Read the model definition and answer for the solid it produces. Units are mm, in the model's axes. A direction names the side the tool comes from. Coordinates: 2 decimals unless noted, no trailing zeros. Write each loop counter-clockwise with the first axis right and the second up, starting at its lowest first coordinate (ties: lowest second). Pieces come first, ordered by that corner, then holes. Notation, with made-up numbers: (87.5, 54.5) -> (111.5, 54.5) arc R36 cw to (111.5, 90.5) -> close; hole circle Ø2 at (67.5, -32.75). An arc over 180 degrees is marked (long way). Use CSV: the item, a comma, the result in double quotes. Start each with the question number.
Autodesk Inventor part; units mm, degrees
ref_plane "YZ Plane" through (0, 0, 0) normal (1, 0, 0) x (0, 1, 0)
ref_plane "XZ Plane" through (0, 0, 0) normal (0, 1, 0) x (-1, 0, 0)
ref_plane "XY Plane" through (0, 0, 0) normal (0, 0, 1) x (1, 0, 0)
sketch "Sketch2" plane through (0, 0, 0) normal (0, 0, 1) x (1, 0, 0)
  circle A0 centre (0, 0) radius 12.7
  dimension "d4" = 25.4
extrude "Extrusion2" add sketch "Sketch2" against normal blind 25.4
chamfer "Chamfer1" distance 1.524 angle 45 1 edges at (-12.7, 0, 0) measured on face at (-3.6254, -0.9542, 0)
sketch "Sketch3" plane through (0, 0, -25.4) normal (0, 0, -1) x (-1, 0, 0)
  circle A0 centre (0, 0) radius 9.144
  dimension "d10" = 18.288
extrude "Extrusion3" add sketch "Sketch3" along normal blind 6.35
sketch "Sketch4" plane through (0, 0, -31.75) normal (0, 0, -1) x (-1, 0, 0)
  circle A0 centre (0, 0) radius 11.049
  dimension "d13" = 22.098
extrude "Extrusion4" add sketch "Sketch4" along normal blind 25.4
thread "Thread1"
chamfer "Chamfer2" distance 1.524 angle 45 1 edges at (11.049, 0, -57.15) measured on face at (-0.3422, 2.8186, -57.15)
sketch "Sketch5" plane through (0, 0, -57.15) normal (0, 0, -1) x (-1, 0, 0)
  circle A0 centre (0, 0) radius 6.477
  dimension "d21" = 12.954
extrude "Extrusion5" add sketch "Sketch5" along normal blind 6.35
sketch "Sketch6" plane through (0, 0, -63.5) normal (0, 0, -1) x (-1, 0, 0)
  circle A0 centre (0, 0) radius 7.874
  dimension "d24" = 15.748
extrude "Extrusion6" add sketch "Sketch6" along normal blind 25.4
thread "Thread2"
chamfer "Chamfer3" distance 1.524 angle 45 1 edges at (7.874, 0, -88.9) measured on face at (-0.2439, 2.0086, -88.9)
sketch "Sketch7" plane through (0, 0, -88.9) normal (0, 0, -1) x (-1, 0, 0)
  circle A0 centre (0, 0) radius 5.461
  dimension "d32" = 10.922
extrude "Extrusion7" add sketch "Sketch7" along normal blind 6.35
sketch "Sketch8" plane through (0, 0, -95.25) normal (0, 0, -1) x (-1, 0, 0)
  circle A0 centre (0, 0) radius 6.35
  dimension "d35" = 12.7
extrude "Extrusion8" add sketch "Sketch8" along normal blind 25.4
thread "Thread3"
chamfer "Chamfer4" distance 1.524 angle 45 1 edges at (6.35, 0, -120.65) measured on face at (1.8127, -0.4771, -120.65)
properties part number "13_3"
1) The mould has two halves that part along Z. Classify faces 4 (the face through (0, 0, 0)), 5 (the face through (1.438, -10.955, -43.521)), 6 (the face through (3, -6, -63.5)), 7 (the face through (0, 0, -120.65)): pulls with the +Z half, pulls with the -Z half, needs draft (parallel to the pull), parting line crosses it, or undercut.
2) Find the intervals of material crossed by line 1 along Z through (x, y) = (7.5, 5.75); line 2 along Y through (x, z) = (-0.5, -60.5); line 3 along Z through (x, y) = (-5.5, -3), in increasing order.
3) Section A-A, the plane z = -99.5 is taken. Give the vertices of the cut face in (x, y), plus the area to 3 significant figures.
4) Which of the six approach directions +Z, -Z, +X, -X, +Y, -Y give full straight-line access (tool end or side, diameter ignored) to faces 1 (the face through (-2.75, -12.4, -13.29)), 2 (the face through (1.38, 6.2, -107.02)), 3 (the face through (1.982, 8.927, -28.531))?
5) Each of these flat-tipped pins is pushed along its axis until it touches: pin 1 (8 mm diameter, centred on x = -8.5, z = -32, fed in from +Y); pin 2 (4 mm diameter, centred on y = 2, z = -55, fed in from +X); pin 3 (15 mm diameter, centred on x = 4.5, y = -3.5, fed in from -Z); pin 4 (2 mm diameter, centred on y = -2, z = -50, fed in from -X). Where does it stop, or does it pass through?
6) Section B-B, the plane z = -26.5 is taken. Give the vertices of the cut face in (x, y), plus the area to 3 significant figures.
The answers:
1,face 4,"pulls with the +Z half"
1,face 5,"needs draft"
1,face 6,"undercut"
1,face 7,"pulls with the -Z half"
2,line 1,"z = -57.15 to -31.75, -25.4 to 0"
2,line 2,"y = -6.46 to 6.46"
2,line 3,"z = -119.21 to -95.25, -88.9 to 0"
3,outline,"circle Ø12.7 at (0, 0)"
3,area,"127 mm^2"
4,face 1,"+Z, -Z"
4,face 2,"-Z"
4,face 3,"none"
5,pin 1,"stops at y = 10.09"
5,pin 2,"stops at x = 11.05"
5,pin 3,"stops at z = -120.65"
5,pin 4,"stops at x = -11"
6,outline,"circle Ø18.29 at (0, 0)"
6,area,"263 mm^2"
